Build history of the part. All positions in model axes, mm. A direction names the side the tool comes from. Round coordinates to 2 decimals unless told otherwise and drop trailing zeros. Order: outer loops, then holes, each group sorted by start corner. A loop starts at its lowest first (then second) coordinate and runs counter-clockwise, first axis right, second up. Notation, with made-up numbers: (-10.75, 13.25) -> (6.25, 13.25) arc R4 ccw to (6.25, 20.25) -> close; hole circle Ø8 at (82.25, 80). An arc over 180 degrees is marked (long way). Use a Markdown table: item, result. Add a question column.
Item 1: Two-plate mould, pull along Y, no slides. Class faces 1 (the face through (22.98, -20.04, -16.79)), 2 (the face through (-19, 8, 0)): released by +Y, released by -Y, zero draft, split by the parting line, or undercut.
Item 2: Slice it at C-C, the plane z = 4.5. Give the cut face in (x, y) (3 decimals), plus the area to 3 significant figures.
Item 3: 3-axis set-ups, long thin cutter, end or side, ignore diameter. For faces 3 (the face through (22.244, 1.502, 4.93)), 4 (the face through (-54.112, -20.035, -30.768)), 5 (the face through (-26, 17.5, -16)), 6 (the face through (-70, 0, 5)): which of +Z, -Z, +X, -X, +Y, -Y reach the whole face in a straight line?
Item 4: Probe L1, parallel to Y at x = -63, z = -23; L2, parallel to Z at x = -38, y = -16; L3, parallel to X at y = -4, z = 3.5 (3 decimals). List the from-to ranges inside material, lowest first.
Item 5: Pin check, flat tips, straight feed: pin 1 (10.5 mm diameter, centred on x = -1.5, y = -0.5, fed in from -Z); pin 2 (5 mm diameter, centred on x = 0, z = -28, fed in from +Y); pin 3 (8 mm diameter, centred on x = -33.5, y = 14, fed in from -Z); pin 4 (5 mm diameter, centred on y = -4, z = 3.5, fed in from -X). Stop position of each tip, or through.
Item 6: Slice it at D-D, the plane z = -21. Give the cut face in (x, y), plus the area to 3 significant figures.
Item 7: Slice it at A-A, the plane z = -38. Give the cut face in (x, y).
Item 8: Slice it at B-B, the plane x = 0. Give the cut face in (y, z).
from build123d import *

# Parameters (mm, degrees)
SKETCH2_W           = 102.74136237
SKETCH2_H           = 45
SKETCH2_R           = 5
BOSS_EXTRUDE1_DEPTH = 10
SKETCH3_R           = 5
SKETCH3_R_2         = 3.96875
BOSS_EXTRUDE2_DEPTH = 5


with BuildPart() as part:
    # Sketch2 → Boss-Extrude1 (new body)
    with BuildSketch(Plane.XY):
        with Locations((-18.629318815, 0)):
            Rectangle(SKETCH2_W, SKETCH2_H)
        with Locations((17.475, 0)):
            Circle(SKETCH2_R, mode=Mode.SUBTRACT)
        with Locations((-17.475, 0)):
            Circle(SKETCH2_R, mode=Mode.SUBTRACT)
    extrude(amount=BOSS_EXTRUDE1_DEPTH)

    # Sketch3 → Boss-Extrude2 (add)
    with BuildSketch(Plane(origin=(0, 22.5, 0), x_dir=(1, 0, 0), z_dir=(0, 1, 0))):
        with BuildLine():
            Line((32.74136237, -10), (32.74136237, 0))
            Line((32.74136237, 0), (12.941825805, 34.051297768))
            ThreePointArc((12.941825805, 34.051297768), (-0.958840285, 41.349241447), (-13.571539602, 32))
            ThreePointArc((-13.571539602, 32), (-30.051797166, 27.060729478), (-47.230652005, 28))
            ThreePointArc((-47.230652005, 28), (-54.208421011, 30.810382158), (-60.996938829, 34.051297768))
            ThreePointArc((-60.996938829, 34.051297768), (-77.438081848, 33.940854804), (-83.493041421, 18.654885879))
            ThreePointArc((-83.493041421, 18.654885879), (-77.649691032, 8.674181664), (-70, 0))
            Line((-70, 0), (-70, -10))
            Line((-70, -10), (32.74136237, -10))
        make_face()
        with Locations(Location((-69.135650368, 21.809953676, 0), (0, 0, 270))):
            Circle(SKETCH3_R, mode=Mode.SUBTRACT)
        with Locations(Location((0, 28, 0), (0, 0, 270))):
            Circle(SKETCH3_R_2, mode=Mode.SUBTRACT)
    boss_extrude2 = extrude(amount=-BOSS_EXTRUDE2_DEPTH)

    # Mirror1: Boss-Extrude2 across plane
    add(boss_extrude2.mirror(Plane.ZX))


solid = part.part
Check sheet entries:
| question | item | result |
|---|---|---|
| 1 | face 1 | zero draft |
| 1 | face 2 | undercut |
| 2 | outline | (-70, -22.5) -> (32.741, -22.5) -> (32.741, 22.5) -> (-70, 22.5) -> close; hole circle Ø10 at (-17.475, 0); hole circle Ø10 at (17.475, 0) |
| 2 | area | 4,470 mm2 |
| 3 | face 3 | +Z, -Z |
| 3 | face 4 | -Z, +Y, -Y |
| 3 | face 5 | -Z, +X, -X |
| 3 | face 6 | +Z, -X, +Y, -Y |
| 4 | L1 | -22.5 to -17.5, 17.5 to 22.5 |
| 4 | L2 | 0 to 10 |
| 4 | L3 | -70 to -20.475, -14.475 to 14.475, 20.475 to 32.741 |
| 5 | pin 1 | z = 0 |
| 5 | pin 2 | through |
| 5 | pin 3 | z = -26.9 |
| 5 | pin 4 | x = -70 |
| 6 | outline | (-83.81, -22.5) -> (-74.07, -22.5) -> (-74.07, -17.5) -> (-83.81, -17.5) -> close; (-83.81, 17.5) -> (-74.07, 17.5) -> (-74.07, 22.5) -> (-83.81, 22.5) -> close; (-64.2, -22.5) -> (20.53, -22.5) -> (20.53, -17.5) -> (-64.2, -17.5) -> close; (-64.2, 17.5) -> (20.53, 17.5) -> (20.53, 22.5) -> (-64.2, 22.5) -> close |
| 6 | area | 945 mm2 |
| 7 | outline | (-9.24, -22.5) -> (9.6, -22.5) -> (9.6, -17.5) -> (-9.24, -17.5) -> close; (-9.24, 17.5) -> (9.6, 17.5) -> (9.6, 22.5) -> (-9.24, 22.5) -> close |
| 8 | outline | (-22.5, -41.39) -> (-17.5, -41.39) -> (-17.5, -31.97) -> (-22.5, -31.97) -> close; (-22.5, -24.03) -> (-17.5, -24.03) -> (-17.5, 0) -> (17.5, 0) -> (17.5, -24.03) -> (22.5, -24.03) -> (22.5, 10) -> (-22.5, 10) -> close; (17.5, -41.39) -> (22.5, -41.39) -> (22.5, -31.97) -> (17.5, -31.97) -> close |
